Answer from the drawing. Dimensions are ordinates in mm from the lowest x, y and z of the part. Round coordinates to 2 decimals unless told otherwise and drop trailing zeros. Write each loop counter-clockwise with the first axis right and the second up, starting at its lowest first coordinate (ties: lowest second). Pieces come first, ordered by that corner, then holes. Notation, with made-up numbers: (46, 42.25) - (73, 42.25) arc R20 cw to (73, 55.25) - close; hole circle Ø6 at (-18, 26.5). An arc over 180 degrees is marked (long way). One line per item, written item: value. Start each with the question number.
(1) Flat-ended cylindrical pins translate along their axes: pin 1 Ø1.3 at (x, z) = (35.5, 6.3) entering from -Y; pin 2 Ø1.4 at (x, z) = (43.5, 14.3) entering from +Y. Find the tip coordinate at first contact, or state that the pin passes through.
(2) A cutting plane is placed at A-A, the plane z = 23.75. Determine the outline of the cut face in (x, y).
(3) A cutting plane is placed at B-B, the plane x = 8.5. Determine the outline of the cut face in (y, z), plus the area to 3 significant figures.
(4) A cutting plane is placed at C-C, the plane z = 16.5. Determine the outline of the cut face in (x, y), plus the area to 3 significant figures.
(5) Find the intervals of material crossed by L1, parallel to Z at x = 35.5, y = 35.2; L2, parallel to X at y = 33.95, z = 22.3; L3, parallel to Y at x = 5.5, z = 14.5, in increasing order.
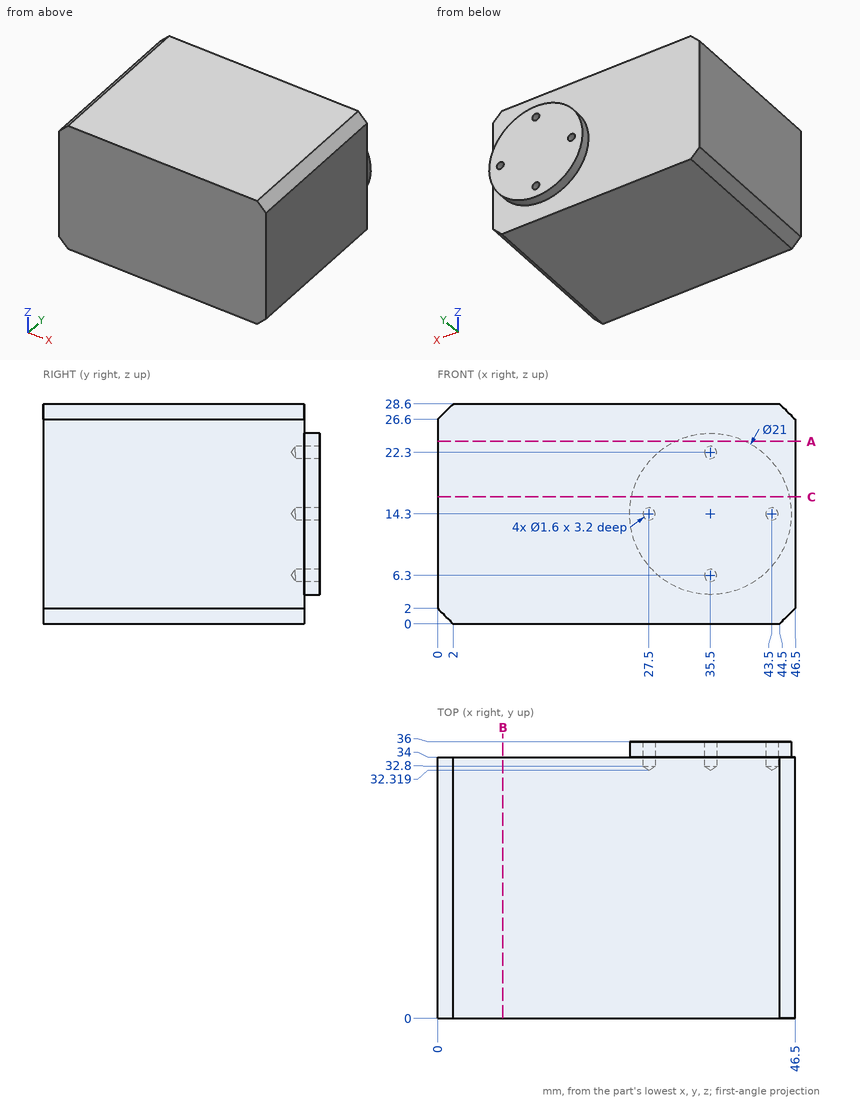
Here are the results:
1. pin 1: y = 0
1. pin 2: y = 32.74
2. outline: (0, 0) - (46.5, 0) - (46.5, 34) - (40.08, 34) - (40.08, 36) - (30.92, 36) - (30.92, 34) - (0, 34) - close
3. outline: (0, 0) - (34, 0) - (34, 28.6) - (0, 28.6) - close
3. area: 972 mm²
4. outline: (0, 0) - (46.5, 0) - (46.5, 34) - (45.77, 34) - (45.77, 36) - (25.23, 36) - (25.23, 34) - (0, 34) - close
4. area: 1,620 mm²
5. L1: 3.8 to 5.5, 7.1 to 21.5, 23.1 to 24.8
5. L2: 0 to 34.7, 36.3 to 46.5
5. L3: 0 to 34
